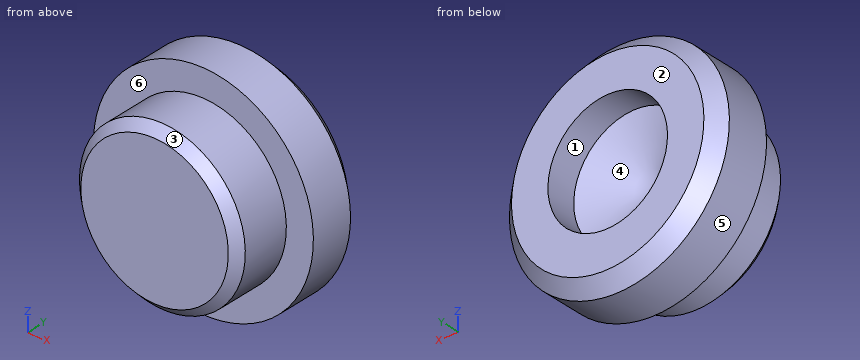
from build123d import *

# Parameters (mm, degrees)
SKETCH1_R           = 4.5974
BOSS_EXTRUDE1_DEPTH = 3.175
SKETCH2_R           = 6.096
BOSS_EXTRUDE2_DEPTH = 3.175
CHAMFER1_SIZE       = 0.762
CHAMFER2_SIZE       = 0.508
SKETCH3_R           = 3.3147
CUT_EXTRUDE1_DEPTH  = 1.6764


with BuildPart() as part:
    # Sketch1 → Boss-Extrude1 (new body)
    with BuildSketch(Plane(origin=(0, 0, 0), x_dir=(1, 0, 0), z_dir=(0, 1, 0))):
        with Locations(Location((0, 0, 0), (0, 0, 270))):
            Circle(SKETCH1_R)
    extrude(amount=BOSS_EXTRUDE1_DEPTH)

    # Sketch2 → Boss-Extrude2 (add)
    with BuildSketch(Plane(origin=(0, 3.175, 0), x_dir=(1, 0, 0), z_dir=(0, 1, 0))):
        with Locations(Location((0, 0, 0), (0, 0, 270))):
            Circle(SKETCH2_R)
    extrude(amount=BOSS_EXTRUDE2_DEPTH)

    # Chamfer1
    chamfer1_edges = [part.edges().sort_by_distance(p)[0] for p in [
        (0, 6.35, -6.096),
    ]]
    chamfer(chamfer1_edges, length=CHAMFER1_SIZE)

    # Chamfer2
    chamfer2_edges = [part.edges().sort_by_distance(p)[0] for p in [
        (0, 0, -4.5974),
    ]]
    chamfer(chamfer2_edges, length=CHAMFER2_SIZE)

    # Sketch3 → Cut-Extrude1 (cut)
    with BuildSketch(Plane(origin=(0, 6.35, 0), x_dir=(1, 0, 0), z_dir=(0, 1, 0))):
        with Locations(Location((0, 0, 0), (0, 0, 270))):
            Circle(SKETCH3_R)
    extrude(amount=-CUT_EXTRUDE1_DEPTH, mode=Mode.SUBTRACT)

    # Cut-Extrude2 cone 1 section (through the dimple's axis) → Cut-Extrude2 (revolve, cut)
    with BuildSketch(Plane(origin=(0, 4.6736, 0), x_dir=(0, 0, 1), z_dir=(1, 0, 0))):
        Polygon((0, 0), (3.3147, 0), (0, 1.339225731), align=None)
    revolve(axis=Axis((0, 4.6736, 0), (0, -1, 0)), mode=Mode.SUBTRACT)


solid = part.part
Can you work these out from the model? Positions are in its coordinate system, mm. Face numbers are marked on the shaded views. A direction names the side the tool comes from. Round coordinates to 2 decimals unless told otherwise and drop trailing zeros. Loops run counter-clockwise (first coordinate to the right, second up) from the corner with the lowest first, then second, coordinate; pieces in that order, holes last. Notation, with made-up numbers: (2, 69.25) - (7, 69.25) arc R4 ccw to (7, 76.25) - close; hole circle Ø5 at (88, -36.5). An arc over 180 degrees is marked (long way). Answer in a Markdown table with one row per item. Add a question column.
Q1. I want a section at A-A on y = 2.75. List the corners of the cut face in (x, z) for me, and give its area (3 significant figures).
Q2. Which directions (+Z, -Z, +X, -X, +Y, -Y) give clear straight access to the entire face, cutting with the end or side of a thin tool? Please do the marked faces 5 and 6.
Q3. I want a section at C-C on y = 3.5. List the corners of the cut face in (x, z) for me.
Q4. I want a section at B-B on y = 4.5. List the corners of the cut face in (x, z) for me, and give its area (3 significant figures).
Q5. For pin 1 Ø2 at (y, z) = (1, -3) entering from +X; pin 2 Ø1.5 at (x, y) = (-4, 2) entering from +Z; pin 3 Ø5.5 at (x, z) = (0, 0) entering from +Y, each with a flat end and sliding along its axis, tell me the tip position at first contact or that it passes through.
Q6. We'd pull the mould along X, two halves only. Please class the marked faces 1, 2, 3 and 4: pulls with the +X half, pulls with the -X half, needs draft (parallel to the pull), parting line crosses it, or undercut.
Q7. I need wall thicknesses on L1, parallel to X at y = 6.05, z = 0; L2, parallel to X at y = 5, z = 0.25; L3, parallel to Z at x = -2.5, y = 5.75. Which ranges of each line are inside material? Lowest first, please.
A:
| question | item | result |
|---|---|---|
| 1 | outline | circle Ø9.19 at (0, 0) |
| 1 | area | 66.4 mm^2 |
| 2 | face 5 | +Y, -Y |
| 2 | face 6 | -Y |
| 3 | outline | circle Ø12.19 at (0, 0); hole circle Ø0.82 at (0, 0) |
| 4 | outline | circle Ø12.19 at (0, 0); hole circle Ø5.77 at (0, 0) |
| 4 | area | 90.6 mm^2 |
| 5 | pin 1 | x = 4.14 |
| 5 | pin 2 | z = 3.25 |
| 5 | pin 3 | y = 4.45 |
| 6 | face 1 | undercut |
| 6 | face 2 | needs draft |
| 6 | face 3 | parting line crosses it |
| 6 | face 4 | undercut |
| 7 | L1 | -5.63 to -3.31, 3.31 to 5.63 |
| 7 | L2 | -6.09 to -3.31, 3.31 to 6.09 |
| 7 | L3 | -5.38 to -2.18, 2.18 to 5.38 |
